Check sheet for the modelled part. Datum: model origin and axes. Units: mm. A direction names the side the tool comes from. Coordinates: 2 decimals unless noted, no trailing zeros. Write each loop counter-clockwise with the first axis right and the second up, starting at its lowest first coordinate (ties: lowest second). Pieces come first, ordered by that corner, then holes. Notation, with made-up numbers: M -0.5,-28.75 L 26.5,-28.75 A19 ccw 26.5,-12.75 Z; hole C 43.5,-9 d4. An arc over 180 degrees is marked long. Answer as CSV lines item,"result". Start each with the question number.
Q1. Access from +Z, -Z, +X, -X, +Y, -Y to the whole of each face (thin tool, end or side, straight path). Record for faces 5 (the flat face through (-8, -39, 1)), 6 (the flat face through (0, -15, 0)).
Q2. Mould release check, pull along Y, two halves, no side actions. Record for faces 1 (the cylindrical face through (-0.62, 17.49, 1.48)), 2 (the flat face through (8, -39, 1)), 3 (the cylindrical face through (11.3, -8.3, 1.5)), 4 (the cylindrical face through (-8.54, -16.1, 1.48)): pulls with the +Y half, pulls with the -Y half, needs draft (parallel to the pull), parting line crosses it, or undercut.
Q3. Sectioned sample at D-D, the plane y = -47.5. Record the cut outline in (x, z).
Q4. Sectioned sample at B-B, the plane y = 0. Record the cut outline in (x, z).
Q5. Thickness scan on line 1 along Y through (x, z) = (0, 2.05); line 2 along Y through (x, z) = (0.5, 2); line 3 along X through (y, z) = (-30, 1.55). Record the ranges inside material, lowest first. Write a range as from..to.
Q6. Sectioned sample at A-A, the plane x = 0. Record the cut outline in (y, z), then the cut area to 3 significant figures.
Q7. Depth check by flat-ended pin: pin 1 Ø1.9 at (x, y) = (0, 13.5) entering from +Z; pin 2 Ø1 at (y, z) = (-18, 1) entering from +X; pin 3 Ø1.5 at (x, z) = (-6, 1.5) entering from -Y; pin 4 Ø0.9 at (y, z) = (-31, 1.5) entering from -X. Enter the tip coordinate at first touch or a pass-through.
Q8. Sectioned sample at C-C, the plane z = 2.15. Record the cut outline in (x, y).
from build123d import *

# Parameters (mm, degrees)
SKETCH_1_R      = 1.6
SKETCH_1_R_2    = 6
SKETCH_1_R_3    = 5
EXTRUDE_1_DEPTH = 3


with BuildPart() as part:
    # 草图1 → 凸台-拉伸1 (new body)
    with BuildSketch(Plane.XY):
        with BuildLine():
            Line((-8, -60), (-8, -18.364367672))
            ThreePointArc((-8, -18.364367672), (-8.559029135, -16.067026214), (-10.111111111, -14.283397078))
            ThreePointArc((-10.111111111, -14.283397078), (0, 17.5), (10.111111111, -14.283397078))
            ThreePointArc((10.111111111, -14.283397078), (8.559029135, -16.067026214), (8, -18.364367672))
            Line((8, -18.364367672), (8, -60))
            ThreePointArc((8, -60), (0, -68), (-8, -60))
        make_face()
        with Locations((0, 13.5)):
            Circle(SKETCH_1_R, mode=Mode.SUBTRACT)
        with Locations((11.691342951, -6.75)):
            Circle(SKETCH_1_R, mode=Mode.SUBTRACT)
        with Locations((-11.691342951, -6.75)):
            Circle(SKETCH_1_R, mode=Mode.SUBTRACT)
        Circle(SKETCH_1_R_2, mode=Mode.SUBTRACT)
        with Locations((0, -60)):
            Circle(SKETCH_1_R_3, mode=Mode.SUBTRACT)
    extrude(amount=EXTRUDE_1_DEPTH)


solid = part.part
Output:
1,face 5,"+Z, -Z, -X, -Y"
1,face 6,"-Z, +X, -X, +Y, -Y"
2,face 1,"parting line crosses it"
2,face 2,"needs draft"
2,face 3,"undercut"
2,face 4,"pulls with the -Y half"
3,outline,"M -8,0 L 8,0 L 8,3 L -8,3 Z"
4,outline,"M -17.5,0 L -6,0 L -6,3 L -17.5,3 Z; M 6,0 L 17.5,0 L 17.5,3 L 6,3 Z"
5,line 1,"y = -68..-65, -55..-6, 6..11.9, 15.1..17.5"
5,line 2,"y = -67.98..-64.97, -55.03..-5.98, 5.98..11.98, 15.02..17.49"
5,line 3,"x = -8..8"
6,outline,"M -68,0 L -65,0 L -65,3 L -68,3 Z; M -55,0 L -6,0 L -6,3 L -55,3 Z; M 6,0 L 11.9,0 L 11.9,3 L 6,3 Z; M 15.1,0 L 17.5,0 L 17.5,3 L 15.1,3 Z"
6,area,"181 mm^2"
7,pin 1,"passes through"
7,pin 2,"stops at x = 8.08"
7,pin 3,"stops at y = -66.04"
7,pin 4,"stops at x = -8"
8,outline,"M -10.11,-14.28 A5 cw -8,-18.36 L -8,-60 A8 ccw 8,-60 L 8,-18.36 A5 cw 10.11,-14.28 A17.5 ccw long Z; hole C -11.69,-6.75 d3.2; hole C 0,0 d12; hole C 0,-60 d10; hole C 0,13.5 d3.2; hole C 11.69,-6.75 d3.2"
